Read the model definition and answer for the solid it produces. Units are mm, in the model's axes. Face numbers are marked on the shaded views. Give positions to 0.01 mm unless a question says otherwise; leave off trailing zeros. Loops run counter-clockwise (first coordinate to the right, second up) from the corner with the lowest first, then second, coordinate; pieces in that order, holes last. Notation, with made-up numbers: (-33.5, 84) - (-21.5, 84) arc R13 ccw to (-21.5, 90) - close; hole circle Ø8 at (43, 20.5). An arc over 180 degrees is marked (long way). Write item = value, one per line.
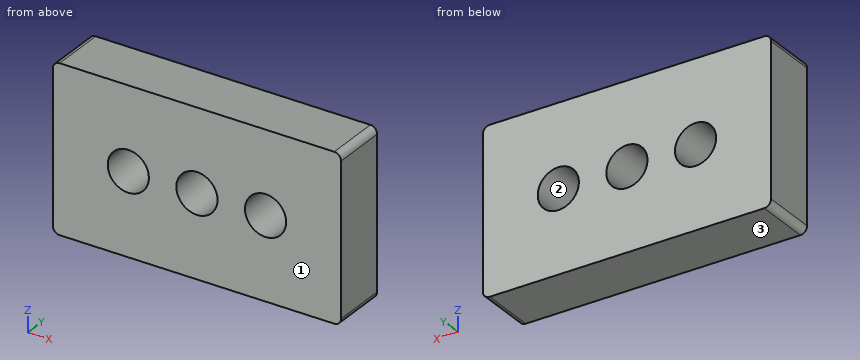
```python
from build123d import *

# Parameters (mm, degrees)
F0_W     = 266.7
F0_H     = 152.4
F1_DEPTH = 50.8
F2_R     = 19.05
F3_DEPTH = 76.2
F4_R     = 6.35


with BuildPart() as f1:
    # F0 (on Front) → F1 (new body)
    with BuildSketch(Plane.XZ):
        Rectangle(F0_W, F0_H)
    extrude(amount=F1_DEPTH)

    # F2 (on face) → F3 (cut)
    with BuildSketch(Plane.XZ.offset(50.8)):
        with BuildLine():
            ThreePointArc((-19.05, 0), (0, -19.05), (19.05, 0))
            ThreePointArc((19.05, 0), (0, 19.05), (-19.05, 0))
        make_face()
        with Locations((-63.5, 0)):
            Circle(F2_R)
        with BuildLine():
            ThreePointArc((82.55, 0), (63.5, 19.05), (44.45, 0))
            ThreePointArc((44.45, 0), (63.5, -19.05), (82.55, 0))
        make_face()
    extrude(amount=-F3_DEPTH, mode=Mode.SUBTRACT)

    # F4
    f4_edges = [f1.edges().sort_by_distance(p)[0] for p in [
        (133.35, -25.4, 76.2),
        (133.35, -25.4, -76.2),
        (-133.35, -25.4, 76.2),
        (-133.35, -25.4, -76.2),
    ]]
    fillet(f4_edges, radius=F4_R)


solid = f1.part
```
1) This flat-tipped pin is pushed along its axis until it touches: P1, Ø23, axis at x = 63.5, z = 0, coming from the +Y side. Where does it stop, or does it pass through?
Output:
P1 = through
2) A cutting plane is placed at B-B on z = 0. Determine the outline of the cut face in (x, y).
Output:
outline = (-133.35, -50.8) - (-82.55, -50.8) - (-82.55, 0) - (-133.35, 0) - close; (-44.45, -50.8) - (-19.05, -50.8) - (-19.05, 0) - (-44.45, 0) - close; (19.05, -50.8) - (44.45, -50.8) - (44.45, 0) - (19.05, 0) - close; (82.55, -50.8) - (133.35, -50.8) - (133.35, 0) - (82.55, 0) - close
3) Find the intervals of material crossed by probe 1 along Z at (x, y) = (0, -22.5); probe 2 along X at (y, z) = (-41, -12.5); probe 3 along X at (y, z) = (-35.5, -17), in increasing order.
Output:
probe_1 = -76.2 to -19.05, 19.05 to 76.2
probe_2 = -133.35 to -77.88, -49.12 to -14.38, 14.38 to 49.12, 77.88 to 133.35
probe_3 = -133.35 to -72.1, -54.9 to -8.6, 8.6 to 54.9, 72.1 to 133.35
4) A cutting plane is placed at C-C on y = -29.5. Determine the outline of the cut face in (x, z), then the cut area to 3 significant figures.
Output:
outline = (-133.35, -69.85) arc R6.35 ccw to (-127, -76.2) - (127, -76.2) arc R6.35 ccw to (133.35, -69.85) - (133.35, 69.85) arc R6.35 ccw to (127, 76.2) - (-127, 76.2) arc R6.35 ccw to (-133.35, 69.85) - close; hole circle Ø38.1 at (-63.5, 0); hole circle Ø38.1 at (0, 0); hole circle Ø38.1 at (63.5, 0)
area = 37,200 mm²
5) A cutting plane is placed at A-A on x = -63.5. Determine the outline of the cut face in (y, z), then the cut area to 3 significant figures.
Output:
outline = (-50.8, -76.2) - (0, -76.2) - (0, -19.05) - (-50.8, -19.05) - close; (-50.8, 19.05) - (0, 19.05) - (0, 76.2) - (-50.8, 76.2) - close
area = 5,810 mm²
6) A cutting plane is placed at D-D on x = 6. Determine the outline of the cut face in (y, z).
Output:
outline = (-50.8, -76.2) - (0, -76.2) - (0, -18.08) - (-50.8, -18.08) - close; (-50.8, 18.08) - (0, 18.08) - (0, 76.2) - (-50.8, 76.2) - close
7) The mould has two halves that part along Z. Classify the marked faces 1, 2 and 3: pulls with the +Z half, pulls with the -Z half, needs draft (parallel to the pull), parting line crosses it, or undercut.
Output:
face_1 = needs draft
face_2 = undercut
face_3 = pulls with the -Z half
